Verification items for the finished model (mm, model axes). A direction names the side the tool comes from. Give positions to 0.01 mm unless a question says otherwise; leave off trailing zeros. Loops run counter-clockwise (first coordinate to the right, second up) from the corner with the lowest first, then second, coordinate; pieces in that order, holes last. Notation, with made-up numbers: (-21.5, -9) - (-10.5, -9) arc R18 ccw to (-10.5, 12) - close; hole circle Ø9 at (1.25, 50). An arc over 180 degrees is marked (long way). One line per question, with ' | ' between items. Start each with the question number.
1. Tool access check on faces 1 (the face through (0, 8, 10)), 2 (the face through (11, 9.865, 33)), 3 (the face through (10, 6.005, 20)). Record the directions out of +Z, -Z, +X, -X, +Y, -Y that give a thin tool (end or side, any length) a straight path to the whole face; none if there is none.
2. Section check A-A, the plane x = 20. Enter the section's corners in (y, z), then the cut area to 3 significant figures.
3. Thickness scan on line 1 along Y through (x, z) = (8.7, -3.35); line 2 along Y through (x, z) = (30.5, -4); line 3 along X through (y, z) = (5, 20). Record the ranges inside material, lowest first. Write a range as from..to.
4. Section check D-D, the plane y = 3. Enter the section's corners in (x, z), then the cut area to 3 significant figures.
5. Depth check by flat-ended pin: pin 1 Ø1.5 at (y, z) = (11.5, 19) entering from +X; pin 2 Ø4.5 at (x, y) = (8.7, 18.56) entering from +Z; pin 3 Ø1 at (x, z) = (36, 6) entering from +Y; pin 4 Ø15 at (x, z) = (19, 19) entering from +Y. Enter the tip coordinate at first touch or a pass-through.
6. Mould release check, pull along Z, two halves, no side actions. Record for faces 4 (the face through (7.35, 40.13, -2.92)), 5 (the face through (5.357, 7.962, 16.748)), 6 (the face through (20, 30, 0)): +Z half, -Z half, draft (parallel to the pull), parting line (faces both ways), or undercut.
7. Section check C-C, the plane z = 20. Enter the section's corners in (x, y), then the cut area to 3 significant figures.
8. Section check B-B, the plane y = 41.16. Enter the section's corners in (x, z).
from build123d import *

# Parameters (mm, degrees)
SKETCH1_W           = 40
SKETCH1_H           = 40
BOSS_EXTRUDE1_DEPTH = 9.864848297
SKETCH2_R           = 15
CUT_EXTRUDE1_DEPTH  = 3.86
SKETCH3_R           = 9.5
CUT_EXTRUDE2_DEPTH  = 2
SKETCH4_R           = 3.05
CUT_EXTRUDE3_DEPTH  = 57.871254602
SKETCH5_W           = 40
SKETCH5_H           = 5.913501164
BOSS_EXTRUDE3_DEPTH = 49.86
SKETCH7_R           = 1.7
CUT_EXTRUDE4_DEPTH  = 76.40570005
FILLET2_R           = 1


with BuildPart() as part:
    # Sketch1 → Boss-Extrude1 (new body)
    with BuildSketch(Plane(origin=(0, 0, 0), x_dir=(1, 0, 0), z_dir=(0, 1, 0))):
        with Locations((20, -20)):
            Rectangle(SKETCH1_W, SKETCH1_H)
    extrude(amount=BOSS_EXTRUDE1_DEPTH)

    # Sketch2 → Cut-Extrude1 (cut)
    with BuildSketch(Plane(origin=(0, 9.864848297, 0), x_dir=(1, 0, 0), z_dir=(0, 1, 0))):
        with Locations(Location((20, -20, 0), (0, 0, 270))):
            Circle(SKETCH2_R)
    extrude(amount=-CUT_EXTRUDE1_DEPTH, mode=Mode.SUBTRACT)

    # Sketch3 → Cut-Extrude2 (cut)
    with BuildSketch(Plane(origin=(0, 6.004848297, 0), x_dir=(1, 0, 0), z_dir=(0, 1, 0))):
        with Locations(Location((20, -20, 0), (0, 0, 270))):
            Circle(SKETCH3_R)
    extrude(amount=-CUT_EXTRUDE2_DEPTH, mode=Mode.SUBTRACT)

    # Sketch4 → Cut-Extrude3 (cut, through all)
    with BuildSketch(Plane(origin=(0, 4.004848297, 0), x_dir=(1, 0, 0), z_dir=(0, 1, 0))):
        with Locations(Location((20, -20, 0), (0, 0, 270))):
            Circle(SKETCH4_R)
    extrude(amount=-CUT_EXTRUDE3_DEPTH, mode=Mode.SUBTRACT)

    # Sketch5 → Boss-Extrude3 (add)
    with BuildSketch(Plane(origin=(0, 0, 0), x_dir=(1, 0, 0), z_dir=(0, 1, 0))):
        with Locations((20, 2.956750582)):
            Rectangle(SKETCH5_W, SKETCH5_H)
    extrude(amount=BOSS_EXTRUDE3_DEPTH)

    # Sketch7 → Cut-Extrude4 (cut, through all)
    with BuildSketch(Plane.XY):
        with Locations((8.7, 18.564848297)):
            Circle(SKETCH7_R)
        with Locations((31.3, 18.564848297)):
            Circle(SKETCH7_R)
        with Locations((31.3, 41.16)):
            Circle(SKETCH7_R)
        with Locations((8.7, 41.16)):
            Circle(SKETCH7_R)
    extrude(amount=-CUT_EXTRUDE4_DEPTH, mode=Mode.SUBTRACT)

    # Fillet2
    fillet2_edges = [part.edges().sort_by_distance(p)[0] for p in [
        (20, 9.864848297, 0),
    ]]
    fillet(fillet2_edges, radius=FILLET2_R)


solid = part.part
Results list:
1) face 1: +Z, -Z, -X, +Y, -Y | face 2: +Z, +X, -X, +Y | face 3: +Y
2) outline: (0, -5.91) - (49.86, -5.91) - (49.86, 0) - (10.86, 0) arc R1 cw to (9.86, 1) - (9.86, 5) - (6, 5) - (6, 10.5) - (4, 10.5) - (4, 16.95) - (0, 16.95) - close; (0, 23.05) - (4, 23.05) - (4, 29.5) - (6, 29.5) - (6, 35) - (9.86, 35) - (9.86, 40) - (0, 40) - close | area: 511 mm²
3) line 1: 0..16.86, 20.26..39.46, 42.86..49.86 | line 2: 0..17.06, 20.06..39.66, 42.66..49.86 | line 3: 0..10.5, 29.5..40
4) outline: (0, -5.91) - (40, -5.91) - (40, 40) - (0, 40) - close; hole circle Ø6.1 at (20, 20) | area: 1,810 mm²
5) pin 1: through | pin 2: z = 0 | pin 3: y = 9.86 | pin 4: y = 4
6) face 4: draft | face 5: undercut | face 6: +Z half
7) outline: (0, 0) - (16.95, 0) - (16.95, 4) - (10.5, 4) - (10.5, 6) - (5, 6) - (5, 9.86) - (0, 9.86) - close; (23.05, 0) - (40, 0) - (40, 9.86) - (35, 9.86) - (35, 6) - (29.5, 6) - (29.5, 4) - (23.05, 4) - close | area: 216 mm²
8) outline: (0, -5.91) - (7, -5.91) - (7, 0) - (0, 0) - close; (10.4, -5.91) - (29.6, -5.91) - (29.6, 0) - (10.4, 0) - close; (33, -5.91) - (40, -5.91) - (40, 0) - (33, 0) - close
